from build123d import *

# Parameters (mm, degrees)
F1_DEPTH  = 25.4
F2_DEPTH  = 50.8
F5_DEPTH  = 25.4
F6_DEPTH  = 4.572
F8_DEPTH  = 4.826
F9_R      = 2.841234
F10_DEPTH = 49.784


with BuildPart() as f1:
    # F0 (on Top) → F1 (new body)
    with BuildSketch(Plane.XY):
        with BuildLine():
            Line((-36.646917, 10.717721), (-36.646917, 17.666442))
            ThreePointArc((-36.646917, 17.666442), (-50.079254, 4.234106), (-36.646917, -9.19823))
            Line((-36.646917, -9.19823), (-36.646917, -2.249508))
            ThreePointArc((-36.646917, -2.249508), (-43.130532, 4.234106), (-36.646917, 10.717721))
        make_face()
        with BuildLine():
            Line((37.230935, 17.666442), (-36.646917, 17.666442))
            Line((-36.646917, 17.666442), (-36.646917, 10.717721))
            ThreePointArc((-36.646917, 10.717721), (-32.06231, 8.818714), (-30.163303, 4.234106))
            ThreePointArc((-30.163303, 4.234106), (-32.06231, -0.350501), (-36.646917, -2.249508))
            Line((-36.646917, -2.249508), (-36.646917, -9.19823))
            Line((-36.646917, -9.19823), (37.230935, -9.19823))
            Line((37.230935, -9.19823), (37.230935, -2.894706))
            ThreePointArc((37.230935, -2.894706), (30.102123, 4.234106), (37.230935, 11.362918))
            Line((37.230935, 11.362918), (37.230935, 17.666442))
        make_face()
        Polygon((-17.989082, 0), (-17.989082, 9.521575), (21.121064, 9.521575), (21.121064, 0), (21.121064, -3.904298), (-17.989082, -3.904298), align=None, mode=Mode.SUBTRACT)
        with BuildLine():
            ThreePointArc((37.230935, -9.19823), (50.663271, 4.234106), (37.230935, 17.666442))
            Line((37.230935, 17.666442), (37.230935, 11.362918))
            ThreePointArc((37.230935, 11.362918), (42.271766, 9.274937), (44.359747, 4.234106))
            ThreePointArc((44.359747, 4.234106), (42.271766, -0.806725), (37.230935, -2.894706))
            Line((37.230935, -2.894706), (37.230935, -9.19823))
        make_face()
    extrude(amount=F1_DEPTH)

    # F0 (on Top) → F2 (join)
    with BuildSketch(Plane.XY):
        Polygon((21.121064, 9.521575), (-17.989082, 9.521575), (-17.989082, 0), (-17.989082, -3.904298), (21.121064, -3.904298), (21.121064, 0), align=None)
    extrude(amount=F2_DEPTH)

    # F4 (on face) → F5 (cut)
    with BuildSketch(Plane.XZ.offset(3.904298)):
        with BuildLine():
            Line((16.338727, 50.8), (-13.450965, 50.8))
            ThreePointArc((-13.450965, 50.8), (1.443881, 32.607662), (16.338727, 50.8))
        make_face()
    extrude(amount=-F5_DEPTH, mode=Mode.SUBTRACT)

    # F3 (on face) → F6 (join)
    with BuildSketch(Plane(origin=(-17.989082, 0, 0), x_dir=(0, -1, 0), z_dir=(-1, 0, 0))):
        with BuildLine():
            Line((-9.521575, 50.8), (3.904298, 50.8))
            ThreePointArc((3.904298, 50.8), (-2.808638, 57.512936), (-9.521575, 50.8))
        make_face()
    extrude(amount=-F6_DEPTH)

    # F7 (on face) → F8 (join)
    with BuildSketch(Plane.YZ.offset(21.121064)):
        with BuildLine():
            Line((-3.904298, 50.8), (9.521575, 50.8))
            ThreePointArc((9.521575, 50.8), (2.808638, 57.512936), (-3.904298, 50.8))
        make_face()
    extrude(amount=-F8_DEPTH)

    # F9 (on face) → F10 (cut)
    with BuildSketch(Plane(origin=(-17.989082, 0, 0), x_dir=(0, -1, 0), z_dir=(-1, 0, 0))):
        with Locations((-2.808638, 50.8)):
            Circle(F9_R)
    extrude(amount=-F10_DEPTH, mode=Mode.SUBTRACT)


solid = f1.part
The listing builds one solid part. Answer for the finished solid, in the listing's coordinates (mm). A direction names the side the tool comes from. Give positions to 0.01 mm unless a question says otherwise; leave off trailing zeros. Write each loop counter-clockwise with the first axis right and the second up, starting at its lowest first coordinate (ties: lowest second). Pieces come first, ordered by that corner, then holes.
1) Given P1, Ø5, axis at y = 6.5, z = 7, coming from the -X side; P2, Ø12, axis at y = 11.5, z = 44.5, coming from the -X side; P3, Ø6, axis at x = 17.5, y = -6, coming from the +Z side (3 decimals); P4, Ø12.5, axis at x = -7.5, z = 35, coming from the +Y side, each flat-ended and moving along its own axis, determine where each tip first touches the part or whether it passes through.
2) Section D-D (y = -5.5) is taken. Write down the section's boundary in (x, z), and give its area (3 significant figures).
3) Section A-A (z = 45) is taken. Write down the section's boundary in (x, y), and give its area (3 significant figures).
4) Find the intervals of material crossed by L1, parallel to X at y = 3.75, z = 16.5; L2, parallel to Y at x = -16.8, z = 50.8; L3, parallel to X at y = 9.5, z = 15.5, in increasing order.
5) Section B-B (z = 9) is taken. Write down the section's boundary in (x, y), and give its area (3 significant figures).
6) A tool of negligible diameter and unlimited length cuts with its end or side. For faces 5 (the face through (2, 9.522, 32)), 6 (the face through (21.121, 3, 42)), 7 (the face through (1, -3.904, 32)), from which of +Z, -Z, +X, -X, +Y, -Y can it reach the whole face along a straight path? Write none if from no direction.
7) Section C-C (x = 28) is taken. Write down the section's boundary in (y, z).
8) For a pull along X with two mould halves and no side action, classify faces 1 (the face through (1, 17.666, 13)), 2 (the face through (50.66, 3.94, 12.52)), 3 (the face through (-17.989, 3, 42)), 4 (the face through (-13.417, 3, 54)) as pulls with the +X half, pulls with the -X half, needs draft (parallel to the pull), parting line crosses it, or undercut.
Response:
1. P1: stops at x = -50.08
1. P2: stops at x = -17.99
1. P3: stops at z = 54.165
1. P4: stops at y = 9.52
2. outline: (-45.9, 0) - (46.49, 0) - (46.49, 25.4) - (-45.9, 25.4) - close
2. area: 2,350 mm2
3. outline: (-17.99, -3.9) - (-13.49, -3.9) - (-13.49, 9.52) - (-17.99, 9.52) - close; (16.38, -3.9) - (21.12, -3.9) - (21.12, 9.52) - (16.38, 9.52) - close
3. area: 124 mm2
4. L1: x = -50.07 to -43.11, -30.18 to 30.12, 44.34 to 50.65
4. L2: y = -3.9 to -0.03, 5.65 to 9.52
4. L3: x = -49 to -40.43, -32.86 to 32.43, 42.04 to 49.59
5. outline: (-36.65, -9.2) - (37.23, -9.2) arc R13.43 ccw to (37.23, 17.67) - (-36.65, 17.67) arc R13.43 ccw to start; hole (-36.65, 10.72) arc R6.48 ccw (long way) to (-30.16, 4.23) arc R6.48 ccw to start; hole (37.23, -2.89) arc R7.13 ccw to (44.36, 4.23) arc R7.13 ccw to (37.23, 11.36) arc R7.13 ccw to start
5. area: 2,260 mm2
6. face 5: +Z, +X, -X, +Y
6. face 6: +Z, +X, +Y, -Y
6. face 7: +Z, +X, -X, -Y
7. outline: (-9.2, 0) - (17.67, 0) - (17.67, 25.4) - (-9.2, 25.4) - close
8. face 1: needs draft
8. face 2: pulls with the +X half
8. face 3: pulls with the -X half
8. face 4: undercut
